Check sheet for the modelled part. Datum: model origin and axes. Units: mm. Face numbers are marked on the shaded views. A direction names the side the tool comes from. Coordinates: 2 decimals unless noted, no trailing zeros. Write each loop counter-clockwise with the first axis right and the second up, starting at its lowest first coordinate (ties: lowest second). Pieces come first, ordered by that corner, then holes. Notation, with made-up numbers: M 76.5,83.5 L 97.5,83.5 A15 cw 97.5,87.5 Z; hole C -28,30 d1. An arc over 180 degrees is marked long. Answer as CSV lines item,"result". Start each with the question number.
Q1. Sectioned sample at C-C, the plane z = 26.5. Record the cut outline in (x, y), then the cut area to 3 significant figures.
Q2. Sectioned sample at B-B, the plane y = -5.5. Record the cut outline in (x, z), then the cut area to 3 significant figures.
Q3. Sectioned sample at D-D, the plane x = 0.75. Count the separate pieces of the cut face and the enclosed holes in it, then the cut area to 3 significant figures.
Q4. Sectioned sample at A-A, the plane x = 3.5. Record the cut outline in (y, z), then the cut area to 3 significant figures.
Q5. Mould release check, pull along X, two halves, no side actions. Record for the marked faces 1, 2 and 3: pulls with the +X half, pulls with the -X half, needs draft (parallel to the pull), parting line crosses it, or undercut.
Q6. Access from +Z, -Z, +X, -X, +Y, -Y to the whole of each face (thin tool, end or side, straight path). Record for the marked faces 4, 5 and 6.
Q7. Depth check by flat-ended pin: pin 1 Ø4 at (x, z) = (-5, 3.5) entering from -Y; pin 2 Ø1.5 at (y, z) = (-1.5, 24.5) entering from +X; pin 3 Ø1 at (x, z) = (-0.5, 14.5) entering from -Y. Enter the tip coordinate at first touch or a pass-through.
Q8. Thickness scan on line 1 along Z through (x, y) = (-2, -1.25); line 2 along Z through (x, y) = (1.75, -5); line 3 along Y through (x, z) = (0, 0.9). Record the ranges inside material, lowest first. Write a range as from..to.
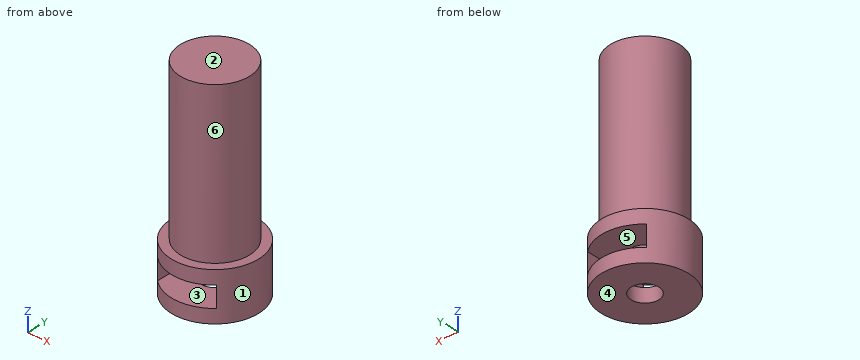
Autodesk Inventor part; units mm, degrees
ref_plane "YZ Plane" through (0, 0, 0) normal (1, 0, 0) x (0, 1, 0)
ref_plane "XZ Plane" through (0, 0, 0) normal (0, 1, 0) x (-1, 0, 0)
ref_plane "XY Plane" through (0, 0, 0) normal (0, 0, 1) x (1, 0, 0)
sketch "Boceto1" plane through (0, 0, 0) normal (0, 0, 1) x (1, 0, 0)
  circle A0 centre (0, 0) radius 8.9
  line L0 (6.2933, -6.2933) -> (-6.2933, -6.2933)
  line L1 (-6.2933, -6.2933) -> (-6.2933, 6.2933)
  line L2 (-6.2933, 6.2933) -> (6.2933, 6.2933)
  line L3 (6.2933, 6.2933) -> (6.2933, -6.2933)
  dimension "d0" = 17.8
  dimension "d1" = 12.5865
  dimension "d2" = 12.5865
sketch "Boceto2" plane through (0, 0, 0) normal (0, 1, 0) x (-1, 0, 0)
  line L0 (6.2933, 0) -> (-6.2933, 0)
  line L1 (-6.2933, 0) -> (-6.2933, 2)
  line L2 (-6.2933, 2) -> (6.2933, 2)
  line L3 (6.2933, 2) -> (6.2933, 0)
  line L4 (-6.2933, 0) -> (6.2933, 0)
  line L5 (6.2933, 0) -> (4.2933, 0)
  line L6 (4.2933, 0) -> (4.2933, 7)
  line L7 (4.2933, 7) -> (6.2933, 7)
  line L8 (6.2933, 7) -> (6.2933, 0)
  line L9 (-6.2933, 0) -> (-4.2933, 0)
  line L10 (-4.2933, 0) -> (-4.2933, 7)
  line L11 (-4.2933, 7) -> (-6.2933, 7)
  line L12 (-6.2933, 7) -> (-6.2933, 0)
  line L13 (-6.2933, 7) -> (6.2933, 7)
  line L14 (6.2933, 7) -> (6.2933, 5)
  line L15 (6.2933, 5) -> (-6.2933, 5)
  line L16 (-6.2933, 5) -> (-6.2933, 7)
  line L17 (0, 7) -> (5, 7)
  line L18 (5, 7) -> (5, 30)
  line L19 (5, 30) -> (0, 30)
  line L20 (0, 30) -> (0, 7)
  line L21 (0, 7) -> (0, 0)
  point P0 (6.2933, 10)
  point P1 (6.2933, 15)
  point P2 (6.2933, 20)
  point P3 (6.2933, 25)
  point P4 (6.2933, 30)
  point P5 (4.2933, 2)
  point P6 (-4.2933, 2)
  point P7 (0, 5)
  point P8 (4.2933, 5)
  point P9 (0, 2)
  point P10 (-4.2933, 5)
  dimension "d5" = 2
  dimension "d28" = 2
  dimension "d29" = 5
  dimension "d30" = 23
revolve "Revolución1" add sketch "Boceto2" angle 360 about axis through (0, 0, 7) along (0, 0, -1) contours L0 L6 L2 L3 | L0 L21 L2 L6 | L2 L6 L15 L8 | L15 L6 L7 L8 | L15 L21 L13 L6 | L13 L20 L19 L18 L7
extrude "Extrusión4" cut sketch "Boceto2" against normal mid plane 20 contours L2 L21 L15 L6 | L2 L10 L15 L21
sketch "Boceto4" plane through (0, 0, 0) normal (0, 0, -1) x (-1, 0, 0)
  circle A0 centre (0, 0) radius 2
  dimension "d34" = 4
extrude "Extrusión5" cut sketch "Boceto4" against normal blind 20
chamfer "Chaflán1" distance 2 angle 45 1 edges at (2, 0, 20)
properties part number "_3DPrint"
Output:
1,outline,"C 0,0 d10"
1,area,"78.5 mm^2"
2,outline,"M -3.06,0 L 3.06,0 L 3.06,2 L -3.06,2 Z; M -3.06,5 L 3.06,5 L 3.06,7 L -3.06,7 Z"
2,area,"24.5 mm^2"
3,separate pieces,"3"
3,enclosed holes,"0"
3,area,"219 mm^2"
4,outline,"M -5.23,0 L 5.23,0 L 5.23,2 L -5.23,2 Z; M -5.23,5 L 5.23,5 L 5.23,7 L 3.57,7 L 3.57,30 L -3.57,30 L -3.57,7 L -5.23,7 Z"
4,area,"206 mm^2"
5,face 1,"parting line crosses it"
5,face 2,"needs draft"
5,face 3,"undercut"
6,face 4,"-Z, +X, -X, +Y, -Y"
6,face 5,"+Y, -Y"
6,face 6,"+Z"
7,pin 1,"stops at y = -5.11"
7,pin 2,"stops at x = 4.94"
7,pin 3,"stops at y = -5"
8,line 1,"z = 0..2, 5..30"
8,line 2,"z = 0..2, 5..7"
8,line 3,"y = -6.29..-2, 2..6.29"
